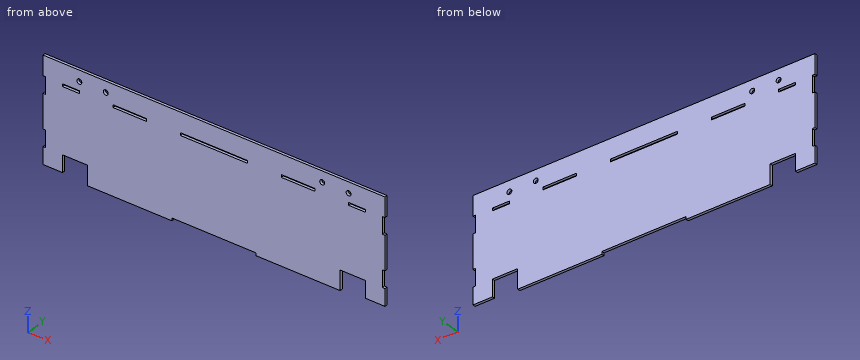
from build123d import *

# Parameters (mm, degrees)
F0_W     = 50
F0_H     = 1.5875
F0_W_2   = 1.5875
F0_H_2   = 20
F0_H_3   = 10
F0_W_3   = 10
F0_R     = 1.4732
F0_W_4   = 20
F0_W_5   = 40
F1_DEPTH = 1.5875


# Not quite as in the source:
# - a length typed as a fraction of an inch, garbled in the dataset ("3 / 203.2 mm" for 3/8 in), is restored


with BuildPart() as f1:
    # F0 (on Front) → F1 (new body)
    with BuildSketch(Plane.XZ):
        with Locations((50, -30.79375)):
            Rectangle(F0_W, F0_H)
        with Locations((-50, -30.79375)):
            Rectangle(F0_W, F0_H)
        with Locations((100.79375, 0)):
            Rectangle(F0_W_2, F0_H_2)
        with Locations((100.79375, -25)):
            Rectangle(F0_W_2, F0_H_3)
        with Locations((-100.79375, 0)):
            Rectangle(F0_W_2, F0_H_2)
        with Locations((-100.79375, -25)):
            Rectangle(F0_W_2, F0_H_3)
        with Locations((100.79375, 25)):
            Rectangle(F0_W_2, F0_H_3)
        with Locations((-100.79375, 25)):
            Rectangle(F0_W_2, F0_H_3)
        Polygon((-100, 30), (100, 30), (101.5875, 30), (101.5875, 31.5875), (-101.5875, 31.5875), (-101.5875, 30), align=None)
        Polygon((100, 20), (100, 30), (-100, 30), (-100, 20), (-100, 10), (-100, -10), (-100, -20), (-100, -30), (-90, -30), (-90, -20), (-75, -20), (-75, -30), (-25, -30), (25, -30), (75, -30), (75, -20), (90, -20), (90, -30), (100, -30), (100, -20), (100, -10), (100, 10), align=None)
        with Locations((-85, 19.20625)):
            Rectangle(F0_W_3, F0_H, mode=Mode.SUBTRACT)
        with Locations((-80, 25.1875)):
            Circle(F0_R, mode=Mode.SUBTRACT)
        with Locations((-64.3028, 25.1875)):
            Circle(F0_R, mode=Mode.SUBTRACT)
        with Locations((-50, 19.20625)):
            Rectangle(F0_W_4, F0_H, mode=Mode.SUBTRACT)
        with Locations((0, 19.20625)):
            Rectangle(F0_W_5, F0_H, mode=Mode.SUBTRACT)
        with Locations((50, 19.20625)):
            Rectangle(F0_W_4, F0_H, mode=Mode.SUBTRACT)
        with Locations((85, 19.20625)):
            Rectangle(F0_W_3, F0_H, mode=Mode.SUBTRACT)
        with Locations((64.3028, 25.1875)):
            Circle(F0_R, mode=Mode.SUBTRACT)
        with Locations((80, 25.1875)):
            Circle(F0_R, mode=Mode.SUBTRACT)
    extrude(amount=F1_DEPTH)


solid = f1.part
Geometry check sheet. Reference: the model listing, model coordinates, mm. Give positions to 0.01 mm unless a question says otherwise; leave off trailing zeros. Loops run counter-clockwise (first coordinate to the right, second up) from the corner with the lowest first, then second, coordinate; pieces in that order, holes last. Notation, with made-up numbers: M 88.5,10 L 134.5,10 A11 cw 134.5,14 Z; hole C 5,-5 d10. An arc over 180 degrees is marked long. Write each question's results on one line, items separated by ' | '.
1) Section check C-C, the plane y = -1.3. Count the separate pieces of the cut face and the enclosed holes in it, plus the area to 3 significant figures.
Answers follow:
separate pieces: 1 | enclosed holes: 9 | area: 12,100 mm2
2) Gauge pin test, flat ends, axial feed: pin 1 (0.5 mm diameter, centred on y = -0.5, z = 15.5, fed in from +X); pin 2 (0.8 mm diameter, centred on x = 83.5, y = -0.5, fed in from -Z). Record the tip position at first contact, or that the pin passes through.
Answers follow:
pin 1: x = 100 | pin 2: z = -20
3) Section check D-D, the plane z = 14.5. Record the boundary of the cut face in (x, y), plus the area to 4 significant figures.
Answers follow:
outline: M -100,-1.59 L 100,-1.59 L 100,0 L -100,0 Z | area: 317.5 mm2
4) Thickness scan on line 1 (X direction, y = -0.15, z = -24); line 2 (Z direction, x = -3, y = -1.2); line 3 (Z direction, x = -88, y = -0.9). Record the ranges inside material, lowest first.
Answers follow:
line 1: -101.59 to -90, -75 to 75, 90 to 101.59 | line 2: -30 to 18.41, 20 to 31.59 | line 3: -20 to 18.41, 20 to 31.59
5) Section check A-A, the plane z = -22.5. Record the boundary of the cut face in (x, y), plus the area to 3 significant figures.
Answers follow:
outline: M -101.59,-1.59 L -90,-1.59 L -90,0 L -101.59,0 Z; M -75,-1.59 L 75,-1.59 L 75,0 L -75,0 Z; M 90,-1.59 L 101.59,-1.59 L 101.59,0 L 90,0 Z | area: 275 mm2
6) Section check B-B, the plane x = 86.5. Record the boundary of the cut face in (y, z), plus the area to 3 significant figures.
Answers follow:
outline: M -1.59,-20 L 0,-20 L 0,18.41 L -1.59,18.41 Z; M -1.59,20 L 0,20 L 0,31.59 L -1.59,31.59 Z | area: 79.4 mm2
